from build123d import *

# Parameters (mm, degrees)
SKETCH1_W           = 20.1
SKETCH1_H           = 35.09
BOSS_EXTRUDE1_DEPTH = 1.6
SKETCH2_R           = 10.05
BOSS_EXTRUDE2_DEPTH = 15
BOSS_EXTRUDE3_DEPTH = 2.65
SKETCH4_W           = 0.64
SKETCH4_H           = 0.64
LPATTERN1_COUNT     = 4
LPATTERN1_PITCH     = 2.5
SKETCH59_R          = 1.5
CUT_EXTRUDE1_DEPTH  = 31.013373788
SKETCH60_R          = 8.375
SKETCH60_R_2        = 4
CUT_EXTRUDE2_DEPTH  = 1.3


with BuildPart() as part:
    # Sketch1 → Boss-Extrude1 (new body)
    with BuildSketch(Plane(origin=(0, 0, 0), x_dir=(1, 0, 0), z_dir=(0, 1, 0))):
        Rectangle(SKETCH1_W, SKETCH1_H)
    extrude(amount=BOSS_EXTRUDE1_DEPTH)

    # Sketch2 → Boss-Extrude2 (add)
    with BuildSketch(Plane(origin=(0, 1.6, 0), x_dir=(1, 0, 0), z_dir=(0, 1, 0))):
        with Locations(Location((0, 7.495, 0), (0, 0, 90))):
            Circle(SKETCH2_R)
    extrude(amount=BOSS_EXTRUDE2_DEPTH)

    # Sketch3 → Boss-Extrude3 (add)
    with BuildSketch(Plane(origin=(0, 1.6, 0), x_dir=(1, 0, 0), z_dir=(0, 1, 0))):
        Polygon((-4.696446609, -14.045), (-2.903575031, -14.045), (-2.550043283, -14.398575031), (-2.550043283, -16.191446609), (-2.903596673, -16.545), (-4.696468251, -16.545), (-5.05, -16.191424969), (-5.05, -14.398553391), align=None)
    boss_extrude3 = extrude(amount=BOSS_EXTRUDE3_DEPTH)

    # Sweep1: sweep along a path in Sketch58
    with BuildLine(Plane.ZY.offset(3.800032462)) as sweep1_path:
        Line((23.97498918, 7.25), (17.47498918, 7.25))
        ThreePointArc((17.47498918, 7.25), (15.707222227, 6.517766953), (14.97498918, 4.75))
        Line((14.97498918, 4.75), (14.97498918, 4.25))
    # Sketch4 → Sweep1 (sweep)
    with BuildSketch(Plane(origin=(0, 4.25, 0), x_dir=(1, 0, 0), z_dir=(0, 1, 0))):
        with Locations((-3.800032462, -15.29498918)):
            Rectangle(SKETCH4_W, SKETCH4_H)
    sweep1 = sweep(path=sweep1_path.line)

    # LPattern1: Boss-Extrude3, Sweep1 ×4
    with Locations(*[(i * LPATTERN1_PITCH, 0, 0) for i in range(1, LPATTERN1_COUNT)]):
        add(boss_extrude3)
        add(sweep1)

    # Sketch59 → Cut-Extrude1 (cut, through all)
    with BuildSketch(Plane(origin=(0, 1.6, 0), x_dir=(1, 0, 0), z_dir=(0, 1, 0))):
        with Locations(Location((-7.5, -14.995, 0), (0, 0, 270))):
            Circle(SKETCH59_R)
        with Locations(Location((7.5, -14.995, 0), (0, 0, 270))):
            Circle(SKETCH59_R)
    extrude(amount=-CUT_EXTRUDE1_DEPTH, mode=Mode.SUBTRACT)

    # Sketch60 → Cut-Extrude2 (cut)
    with BuildSketch(Plane(origin=(0, 16.6, 0), x_dir=(1, 0, 0), z_dir=(0, 1, 0))):
        with Locations(Location((0, 7.495, 0), (0, 0, 270))):
            Circle(SKETCH60_R)
        with Locations(Location((0, 7.495, 0), (0, 0, 270))):
            Circle(SKETCH60_R_2, mode=Mode.SUBTRACT)
    extrude(amount=-CUT_EXTRUDE2_DEPTH, mode=Mode.SUBTRACT)


solid = part.part
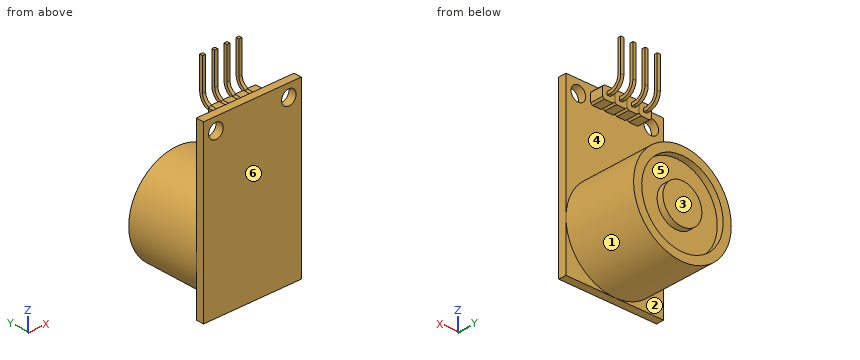
Check sheet for the modelled part. Datum: model origin and axes. Units: mm. Face numbers are marked on the shaded views. A direction names the side the tool comes from. Coordinates: 2 decimals unless noted, no trailing zeros. Write each loop counter-clockwise with the first axis right and the second up, starting at its lowest first coordinate (ties: lowest second). Pieces come first, ordered by that corner, then holes.
Item 1: Cross-section at B-B on z = 13. Record the boundary of the cut face in (x, y), then the cut area to 3 significant figures.
Numbers:
outline: (-10.05, 0) - (10.05, 0) - (10.05, 1.6) - (-10.05, 1.6) - close
area: 32.2 mm2
Item 2: Cross-section at A-A on x = -7.5. Record the boundary of the cut face in (y, z) (3 decimals).
Numbers:
outline: (0, -17.545) - (1.6, -17.545) - (1.6, -14.185) - (16.6, -14.185) - (16.6, -11.222) - (15.3, -11.222) - (15.3, -3.768) - (16.6, -3.768) - (16.6, -0.805) - (1.6, -0.805) - (1.6, 13.495) - (0, 13.495) - close; (0, 16.495) - (1.6, 16.495) - (1.6, 17.545) - (0, 17.545) - close
Item 3: Mould release check, pull along Z, two halves, no side actions. Record for the marked faces 4, 5 and 6: released by +Z, released by -Z, zero draft, split by the parting line, or undercut.
Numbers:
face 4: undercut
face 5: undercut
face 6: zero draft
Item 4: Depth check by flat-ended pin: pin 1 Ø1.4 at (y, z) = (2.5, 15.5) entering from +X; pin 2 Ø3 at (x, z) = (4.5, 11) entering from +Y; pin 3 Ø1.4 at (y, z) = (3, 15.5) entering from -X; pin 4 Ø1.5 at (x, z) = (-1.5, 8) entering from -Y. Enter the tip coordinate at first touch or a pass-through.
Numbers:
pin 1: stops at x = 4.95
pin 2: stops at y = 1.6
pin 3: stops at x = -5.05
pin 4: stops at y = 0
Item 5: Access from +Z, -Z, +X, -X, +Y, -Y to the whole of each face (thin tool, end or side, straight path). Record for the marked faces 1, 2 and 3.
Numbers:
face 1: +Y
face 2: -Z, -X, +Y
face 3: +Z, -Z, +X, -X, +Y
Item 6: Cross-section at D-D on z = -14. Record the boundary of the cut face in (x, y) (3 decimals), then the cut area to 3 significant figures.
Numbers:
outline: (-10.05, 0) - (10.05, 0) - (10.05, 1.6) - (7.661, 1.6) - (7.661, 16.6) - (5.275, 16.6) - (5.275, 15.3) - (-5.275, 15.3) - (-5.275, 16.6) - (-7.661, 16.6) - (-7.661, 1.6) - (-10.05, 1.6) - close
area: 248 mm2
Item 7: Scan lines: probe 1 along Y at (x, z) = (-8, 9.5); probe 2 along Y at (x, z) = (-3.75, -11); probe 3 along Z at (x, y) = (2.25, 0.5) (3 decimals). Record each from-to range of solid material in increasing order.
Numbers:
probe 1: y = 0 to 1.6
probe 2: y = 0 to 15.3
probe 3: z = -17.545 to 17.545
Item 8: Cross-section at C-C on y = 10. Record the boundary of the cut face in (x, z) (3 decimals).
Numbers:
outline: circle Ø20.1 at (0, -7.495)
